from build123d import *

# Parameters (mm, degrees)
EXTRUDE_1_DEPTH    = 40
HOLE_WIZARD_M4_1_D = 3.3


with BuildPart() as part:
    # 草图1 → 凸台-拉伸1 (new body)
    with BuildSketch(Plane(origin=(0, 0, 0), x_dir=(0, 0, -1), z_dir=(1, 0, 0))):
        Polygon((3.464101615, 0), (1.732050808, 3), (-1.732050808, 3), (-3.464101615, 0), (-1.732050808, -3), (1.732050808, -3), align=None)
    extrude(amount=EXTRUDE_1_DEPTH)

    # M4 螺纹孔1 (through all)
    with Locations(Plane.ZY):
        with Locations((0, 0)):
            Hole(HOLE_WIZARD_M4_1_D / 2)


solid = part.part
Part model, mm, in its own coordinate system. Give positions to 0.01 mm unless a question says otherwise; leave off trailing zeros. Write each loop counter-clockwise with the first axis right and the second up, starting at its lowest first coordinate (ties: lowest second). Pieces come first, ordered by that corner, then holes.
1) Cut at A-A on z = 0. Write the cut outline in (x, y), then the cut area to 3 significant figures.
Resolved:
outline: (0, -3) - (40, -3) - (40, -1.65) - (0, -1.65) - close; (0, 1.65) - (40, 1.65) - (40, 3) - (0, 3) - close
area: 108 mm2
2) Cut at D-D on z = -2.75. Write the cut outline in (x, y), then the cut area to 3 significant figures.
Resolved:
outline: (0, -1.24) - (40, -1.24) - (40, 1.24) - (0, 1.24) - close
area: 98.9 mm2
3) Probe L1, parallel to Y at x = 18.5, z = 0; L2, parallel to Z at x = 36.5, y = -0.5; L3, parallel to Z at x = 32, y = -1.5. List the from-to ranges inside material, lowest first.
Resolved:
L1: y = -3 to -1.65, 1.65 to 3
L2: z = -3.18 to -1.57, 1.57 to 3.18
L3: z = -2.6 to -0.69, 0.69 to 2.6
4) Cut at B-B on x = 31. Write the cut outline in (y, z).
Resolved:
outline: (-3, -1.73) - (0, -3.46) - (3, -1.73) - (3, 1.73) - (0, 3.46) - (-3, 1.73) - close; hole circle Ø3.3 at (0, 0)
5) Two-plate mould, pull along Y, no slides. Class faces 1 (the face through (0, 1.4, -1.5)), 2 (the face through (20.28, 1.115, 1.216)), 3 (the face through (20, -3, 0)), 4 (the face through (19.7, 1.5, 2.6)): released by +Y, released by -Y, zero draft, split by the parting line, or undercut.
Resolved:
face 1: zero draft
face 2: undercut
face 3: released by -Y
face 4: released by +Y
6) Cut at C-C on y = 1.25. Write the cut outline in (x, z).
Resolved:
outline: (0, -2.74) - (40, -2.74) - (40, -1.08) - (0, -1.08) - close; (0, 1.08) - (40, 1.08) - (40, 2.74) - (0, 2.74) - close
7) Pin check, flat tips, straight feed: pin 1 (1.5 mm diameter, centred on x = 5, y = 1, fed in from -Z); pin 2 (1 mm diameter, centred on x = 10.5, y = -1.5, fed in from -Z). Stop position of each tip, or through.
Resolved:
pin 1: stops at z = -3.32
pin 2: stops at z = -2.89
